Autodesk Inventor part; units mm, degrees
ref_plane "YZ Plane" through (0, 0, 0) normal (1, 0, 0) x (0, 1, 0)
ref_plane "XZ Plane" through (0, 0, 0) normal (0, 1, 0) x (-1, 0, 0)
ref_plane "XY Plane" through (0, 0, 0) normal (0, 0, 1) x (1, 0, 0)
sketch "Sketch1" plane through (0, 0, 0) normal (0, 0, 1) x (1, 0, 0)
  line L0 (0, 0) -> (100, 0) construction
  arc A0 (10.5, 0) -> (-3.0807, 10.0379) centre (0, 0) ccw construction
  arc A1 (89.5, 0) -> (95.0588, -9.2647) centre (100, 0) ccw construction
  arc A2 (95.0588, -9.2647) -> (60.7485, 1.3948) centre (50, -93.75) ccw
  arc A3 (103.0807, 10.0379) -> (64.7857, 17.3948) centre (50, -162.9167) ccw
  line L1 (35.2143, 17.3948) -> (64.7857, 17.3948)
  line L2 (39.2515, 1.3948) -> (60.7485, 1.3948)
  line L3 (50, 0) -> (50, 2) construction
  line L4 (50, 18) -> (50, 2) construction
  line L5 (35.2143, 17.3948) -> (39.2515, 1.3948) construction
  line L6 (0, 0) -> (37.2329, 9.3948) construction
  arc A4 (39.2515, 1.3948) -> (4.9412, -9.2647) centre (50, -93.75) ccw
  arc A5 (60.7485, 1.3948) -> (39.2515, 1.3948) centre (50, -93.75) ccw construction
  arc A6 (35.2143, 17.3948) -> (-3.0807, 10.0379) centre (50, -162.9167) ccw
  arc A7 (64.7857, 17.3948) -> (35.2143, 17.3948) centre (50, -162.9167) ccw construction
  arc A8 (4.9412, -9.2647) -> (10.5, 0) centre (0, 0) ccw construction
  arc A9 (-3.0807, 10.0379) -> (4.9412, -9.2647) centre (0, 0) ccw
  arc A10 (103.0807, 10.0379) -> (89.5, 0) centre (100, 0) ccw construction
  arc A11 (95.0588, -9.2647) -> (103.0807, 10.0379) centre (100, 0) ccw
  dimension "d0" = 100
  dimension "d1" = 21
  dimension "d2" = 2
  dimension "d3" = 16
  dimension "d30" = 16
  dimension "d31" = 38.3998
extrude "Extrusion1" add sketch "Sketch1" along normal blind 2
sketch "Sketch2" plane through (0, 0, 2) normal (0, 0, 1) x (1, 0, 0)
  line L0 (64.7857, 17.3948) -> (35.2143, 17.3948) construction
  line L1 (39.2515, 1.3948) -> (60.7485, 1.3948) construction
  line L2 (50, 17.3948) -> (50, 1.3948) construction
  line L3 (41, 9.3948) -> (59, 9.3948) construction
  line L4 (46, 6.8448) -> (54, 6.8448)
  line L5 (54, 6.8448) -> (54, 11.9448)
  line L6 (54, 11.9448) -> (46, 11.9448)
  line L7 (46, 11.9448) -> (46, 6.8448)
  line L8 (46, 6.8448) -> (54, 11.9448) construction
  line L9 (54, 6.8448) -> (46, 11.9448) construction
  point P0 (0, 0)
  point P1 (50, 9.3948)
  dimension "d7" = 18
  dimension "d8" = 5.1
  dimension "d9" = 8
extrude "Extrusion2" cut sketch "Sketch2" against normal through all
hole "Hole1" at (41, 9.3948, 2) at (59, 9.3948, 2) direction (0, 0, -1) diameter 2.6 end through all
sketch "Sketch3" plane through (0, 0, 2) normal (0, 0, 1) x (1, 0, 0)
  line L0 (46, 11.9448) -> (54, 11.9448) construction
  line L1 (46, 6.8448) -> (46, 11.9448) construction
  line L2 (54, 6.8448) -> (46, 6.8448) construction
  line L3 (54, 11.9448) -> (54, 6.8448) construction
  line L4 (53.2929, 11.2377) -> (46.7071, 11.2377) construction
  line L5 (46.7071, 11.2377) -> (46.7071, 7.5519) construction
  line L6 (46.7071, 7.5519) -> (53.2929, 7.5519) construction
  line L7 (53.2929, 7.5519) -> (53.2929, 11.2377) construction
  circle A0 centre (46.7071, 11.2377) radius 1
  circle A1 centre (46.7071, 7.5519) radius 1
  circle A2 centre (53.2929, 7.5519) radius 1
  circle A3 centre (53.2929, 11.2377) radius 1
  point P0 (0, 0)
  dimension "d19" = 2
extrude "Extrusion3" cut sketch "Sketch3" against normal through all
sketch "Sketch4" plane through (0, 0, 2) normal (0, 0, 1) x (1, 0, 0)
  arc A0 (95.0588, -9.2647) -> (103.0807, 10.0379) centre (100, 0) ccw construction
  point P0 (0, 0)
  point P1 (0, 0)
hole "Hole2" at (0, 0, 2) at (100, 0, 2) direction (0, 0, -1) diameter 10 end through all
sketch "Sketch5" plane through (0, 0, 2) normal (0, 0, 1) x (1, 0, 0)
  circle A0 centre (0, 0) radius 8 construction
  circle A1 centre (100, 0) radius 5 construction
  circle A2 centre (100, 0) radius 8 construction
  line L0 (-8, 0) -> (0, 0) construction
  line L1 (100, 0) -> (108, 0) construction
  point P0 (-5.6569, -5.6569)
  point P1 (0, -8)
  point P2 (5.6569, -5.6569)
  point P3 (8, 0)
  point P4 (5.6569, 5.6569)
  point P5 (0, 8)
  point P6 (-5.6569, 5.6569)
  point P7 (105.6569, 5.6569)
  point P8 (100, 8)
  point P9 (94.3431, 5.6569)
  point P10 (92, 0)
  point P11 (94.3431, -5.6569)
  point P12 (100, -8)
  point P13 (105.6569, -5.6569)
  dimension "d36" = 16
  dimension "d34" = 360
  dimension "d39" = 360
hole "Hole3" at (-8, 0, 2) at (-5.6569, -5.6569, 2) at (0, -8, 2) at (5.6569, -5.6569, 2) at (8, 0, 2) at (5.6569, 5.6569, 2) at (0, 8, 2) at (-5.6569, 5.6569, 2) at (108, 0, 2) at (105.6569, 5.6569, 2) at (100, 8, 2) at (94.3431, 5.6569, 2) at (92, 0, 2) at (94.3431, -5.6569, 2) at (100, -8, 2) at (105.6569, -5.6569, 2) direction (0, 0, -1) diameter 2.2 end through all
fillet "Fillet1" radius 3 4 edges at (35.2143, 17.3948, 1) (64.7857, 17.3948, 1) (60.7485, 1.3948, 1) (39.2515, 1.3948, 1)
sketch "Sketch6" plane through (0, 0, 2) normal (0, 0, 1) x (1, 0, 0)
  arc A0 (64.9097, 17.3846) -> (64.6624, 17.3948) centre (64.6624, 14.3948) ccw
  line L0 (64.6624, 17.3948) -> (35.3376, 17.3948)
  arc A1 (35.3376, 17.3948) -> (35.0903, 17.3846) centre (35.3376, 14.3948) ccw
  arc A2 (35.0903, 17.3846) -> (-3.0807, 10.0379) centre (50, -162.9167) ccw
  arc A3 (-3.0807, 10.0379) -> (4.9412, -9.2647) centre (0, 0) ccw
  arc A4 (39.0796, 1.3752) -> (4.9412, -9.2647) centre (50, -93.75) ccw
  arc A5 (39.4217, 1.3948) -> (39.0796, 1.3752) centre (39.4217, -1.6052) ccw
  line L1 (39.4217, 1.3948) -> (60.5783, 1.3948)
  arc A6 (60.9204, 1.3752) -> (60.5783, 1.3948) centre (60.5783, -1.6052) ccw
  arc A7 (95.0588, -9.2647) -> (60.9204, 1.3752) centre (50, -93.75) ccw
  arc A8 (95.0588, -9.2647) -> (103.0807, 10.0379) centre (100, 0) ccw
  arc A9 (103.0807, 10.0379) -> (64.9097, 17.3846) centre (50, -162.9167) ccw
  circle A10 centre (100, -8) radius 1.1
  circle A11 centre (92, 0) radius 1.1
  circle A12 centre (100, 8) radius 1.1
  circle A13 centre (108, 0) radius 1.1
  circle A14 centre (0, 8) radius 1.1
  circle A15 centre (8, 0) radius 1.1
  circle A16 centre (0, -8) radius 1.1
  circle A17 centre (-8, 0) radius 1.1
  circle A18 centre (-5.6569, -5.6569) radius 1.1
  circle A19 centre (5.6569, -5.6569) radius 1.1
  circle A20 centre (5.6569, 5.6569) radius 1.1
  circle A21 centre (-5.6569, 5.6569) radius 1.1
  circle A22 centre (105.6569, 5.6569) radius 1.1
  circle A23 centre (94.3431, 5.6569) radius 1.1
  circle A24 centre (94.3431, -5.6569) radius 1.1
  circle A25 centre (105.6569, -5.6569) radius 1.1
  circle A26 centre (0, 0) radius 5
  circle A27 centre (100, 0) radius 5
  arc A28 (52.5858, 6.8448) -> (54, 8.259) centre (53.2929, 7.5519) ccw
  line L2 (52.5858, 6.8448) -> (47.4142, 6.8448)
  arc A29 (46, 8.259) -> (47.4142, 6.8448) centre (46.7071, 7.5519) ccw
  line L3 (46, 8.259) -> (46, 10.5306)
  arc A30 (47.4142, 11.9448) -> (46, 10.5306) centre (46.7071, 11.2377) ccw
  line L4 (47.4142, 11.9448) -> (52.5858, 11.9448)
  arc A31 (54, 10.5306) -> (52.5858, 11.9448) centre (53.2929, 11.2377) ccw
  line L5 (54, 10.5306) -> (54, 8.259)
  circle A32 centre (41, 9.3948) radius 1.3
  circle A33 centre (59, 9.3948) radius 1.3
properties part number "16_013_FEMUR_FRAME_FREE_R1" material "Aluminum 6061"
Input: part model. Units: mm. Frame: model coordinates. A direction names the side the tool comes from. Coordinates: 2 decimals unless noted, no trailing zeros. Loops run counter-clockwise (first coordinate to the right, second up) from the corner with the lowest first, then second, coordinate; pieces in that order, holes last.
(1) Section C-C on z = 1.3. Count the separate pieces of the cut face and the enclosed holes in it, then the cut area to 3 significant figures.
(2) First-contact query: pin 1 Ø1.8 at (x, y) = (100, -8) entering from +Z. Flat tip, straight axial feed; report the tip coordinate or a pass-through.
(3) Set-up query: faces 3 (the face through (54, 9, 1)), 4 (the face through (21.27, -2.41, 0.99)), 5 (the face through (49, 4, 2)). Return all of +Z, -Z, +X, -X, +Y, -Y with unobstructed straight access to the full face (end or side cutting, diameter ignored); none if empty.
(4) Section A-A on x = 41. Return the cut outline in (y, z), then the cut area to 3 significant figures.
(5) Material intervals for probe 1 along X at (y, z) = (-5.5, 1.25); probe 2 along X at (y, z) = (4, 0.3); probe 3 along X at (y, z) = (-7.5, 1), sorted ascending.
(6) Section B-B on x = 100. Return the cut outline in (y, z), then the cut area to 3 significant figures.
(7) Section D-D on x = 8. Return the cut outline in (y, z).
(8) Pull-direction query (X, two-part tool) for faces 1 (the face through (50, 6.845, 1)), 2 (the face through (49, 4, 0)); classes: released by +X, released by -X, zero draft, split by the parting line, or undercut.
Data:
1. separate pieces: 1
1. enclosed holes: 21
1. area: 1,890 mm2
2. pin 1: passes through
3. face 3: +Z, -Z
3. face 4: +Z, -Z, -Y
3. face 5: +Z, +X, -X, +Y, -Y
4. outline: (1.39, 0) - (8.09, 0) - (8.09, 2) - (1.39, 2) - close; (10.69, 0) - (17.39, 0) - (17.39, 2) - (10.69, 2) - close
4. area: 26.8 mm2
5. probe 1: x = -8.94 to -6.75, -4.57 to 4.57, 6.75 to 12.85, 87.15 to 93.25, 95.43 to 104.57, 106.75 to 108.94
5. probe 2: x = -9.71 to -3, 3 to 97, 103 to 109.71
5. probe 3: x = -7.35 to -0.98, 0.98 to 8.42, 91.58 to 99.02, 100.98 to 107.35
6. outline: (-10.5, 0) - (-9.1, 0) - (-9.1, 2) - (-10.5, 2) - close; (-6.9, 0) - (-5, 0) - (-5, 2) - (-6.9, 2) - close; (5, 0) - (6.9, 0) - (6.9, 2) - (5, 2) - close; (9.1, 0) - (10.95, 0) - (10.95, 2) - (9.1, 2) - close
6. area: 14.1 mm2
7. outline: (-7.7, 0) - (-1.1, 0) - (-1.1, 2) - (-7.7, 2) - close; (1.1, 0) - (13.06, 0) - (13.06, 2) - (1.1, 2) - close
8. face 1: undercut
8. face 2: zero draft
